```python
from build123d import *

# Parameters (mm, degrees)
F0_W     = 65.071911
F0_H     = 69.471795
F1_DEPTH = 419.1
F2_R     = 19.622728
F4_D     = 25.4


with BuildPart() as f1:
    # F0 (on Front) → F1 (new body)
    with BuildSketch(Plane.XZ):
        with Locations((32.535956, 80.350911)):
            Rectangle(F0_W, F0_H)
    extrude(amount=F1_DEPTH)

    # F2
    f2_edges = [f1.edges().sort_by_distance(p)[0] for p in [
        (32.535955, -419.1, 115.086809),
    ]]
    fillet(f2_edges, radius=F2_R)

    # F4 (through all)
    with Locations(Plane.XY.offset(115.086809)):
        with Locations((21.306643, -190.605685)):
            Hole(F4_D / 2)


solid = f1.part
```
The model under review builds one solid part; all positions refer to its coordinate system, in mm. Coordinates: 2 decimals unless noted, no trailing zeros. Write each loop counter-clockwise with the first axis right and the second up, starting at its lowest first coordinate (ties: lowest second). Pieces come first, ordered by that corner, then holes.
1) We need section C-C on z = 51.5. State the section outline as (x, y) points.
2) To check wall thickness, follow probe 1 along Y at (x, z) = (26, 72); probe 2 along Y at (x, z) = (14, 54); probe 3 along X at (y, z) = (-198.5, 53) (3 decimals). State the ranges of each line that lie inside material, in increasing order.
3) Clearance check with a flat-ended pin moving along its axis: pin 1 Ø12 at (x, z) = (50.5, 73.5) entering from +Y. State where the tip first meets the part, or that it passes through.
4) The part is to be moulded in two halves that separate along X. For faces 1 (the face through (65.072, -207, 80)), 2 (the face through (32, 0, 81)), 3 (the face through (24.06, -203.004, 79.865)), say which applies: pulls with the +X half, pulls with the -X half, needs draft (parallel to the pull), parting line crosses it, or undercut.
5) We need section A-A on x = 27.5. State the section outline as (y, z) points, then the cut area to 3 significant figures.
6) We need section B-B on z = 99. State the section outline as (x, y) points, then the cut area to 3 significant figures.
Answer list:
1. outline: (0, -419.1) - (65.07, -419.1) - (65.07, 0) - (0, 0) - close; hole circle Ø25.4 at (21.31, -190.61)
2. probe 1: y = -419.1 to -202.41, -178.8 to 0
2. probe 2: y = -419.1 to -200.99, -180.22 to 0
2. probe 3: x = 0 to 11.358, 31.255 to 65.072
3. pin 1: stops at y = 0
4. face 1: pulls with the +X half
4. face 2: needs draft
4. face 3: undercut
5. outline: (-419.1, 45.62) - (-201.69, 45.62) - (-201.69, 115.09) - (-399.48, 115.09) arc R19.62 ccw to (-419.1, 95.46) - close; (-179.52, 45.62) - (0, 45.62) - (0, 115.09) - (-179.52, 115.09) - close
5. area: 27,500 mm2
6. outline: (0, -418.78) - (65.07, -418.78) - (65.07, 0) - (0, 0) - close; hole circle Ø25.4 at (21.31, -190.61)
6. area: 26,700 mm2
